Could you check a few things on this drawing? It's one solid part, dimensions in mm from its lowest x, y, z. Give positions to 0.01 mm unless a question says otherwise; leave off trailing zeros. Order: outer loops, then holes, each group sorted by start corner. A loop starts at its lowest first (then second) coordinate and runs counter-clockwise, first axis right, second up.
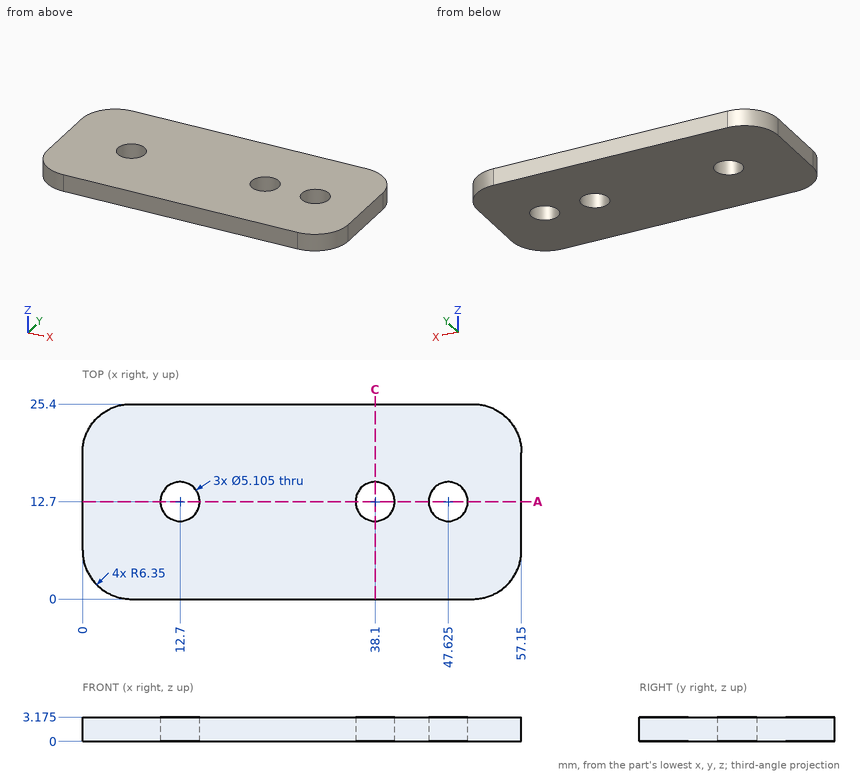
1) Suppose I cut it at A-A (y = 12.7). Give the number of separate pieces and of enclosed holes in the cut face, and give its area (3 significant figures).
2) If I drill on line 1 (Y direction, x = 38.1, z = 1.95); line 2 (Y direction, x = 12.5, z = 2.3) (1 decimal); line 3 (Y direction, x = 54.5, z = 3), over which ranges is the centre line in solid material (lowest first)?
3) Suppose I cut it at C-C (x = 38.1). Please give me the cut outline in (y, z) (1 decimal).
Results:
1. separate pieces: 4
1. enclosed holes: 0
1. area: 133 mm2
2. line 1: y = 0 to 10.15, 15.25 to 25.4
2. line 2: y = 0 to 10.2, 15.2 to 25.4
2. line 3: y = 1.19 to 24.21
3. outline: (0, 0) - (10.1, 0) - (10.1, 3.2) - (0, 3.2) - close; (15.3, 0) - (25.4, 0) - (25.4, 3.2) - (15.3, 3.2) - close
